Read the model definition and answer for the solid it produces. Units are mm, in the model's axes. Coordinates: 2 decimals unless noted, no trailing zeros. Loops run counter-clockwise (first coordinate to the right, second up) from the corner with the lowest first, then second, coordinate; pieces in that order, holes last. Notation, with made-up numbers: M 21.25,79 L 57.25,79 A13 cw 57.25,97 Z; hole C -7,11.25 d3. An arc over 180 degrees is marked long. One line per item, written item: value. Start each with the question number.
1. Flat-ended cylindrical pins translate along their axes: pin 1 (5 mm diameter, centred on y = 56, z = 7, fed in from +X); pin 2 (3 mm diameter, centred on x = 8.5, z = 8, fed in from +Y); pin 3 (3 mm diameter, centred on x = 22, z = 4, fed in from -Y); pin 4 (6 mm diameter, centred on x = 23.5, y = 21, fed in from -Z). Find the tip coordinate at first contact, or state that the pin passes through.
2. The part is cut by section A-A (z = 6.75). Write down the section's boundary in (x, y), then the cut area to 3 significant figures.
3. Consider probe 1 along X at (y, z) = (9.5, 7.25); probe 2 along Y at (x, z) = (23.5, 4.5); probe 3 along X at (y, z) = (19, 0.5). Determine where each line is inside the solid, lowest interval first.
```python
from build123d import *

# Parameters (mm, degrees)
EXTRUDE_1_DEPTH = 10
FILLET_1_R      = 0.5


with BuildPart() as part:
    # 草图1 → 凸台-拉伸1 (new body)
    with BuildSketch(Plane.XY):
        Polygon((0, 75), (37.5, 37.5), (0, 0), align=None)
    extrude(amount=EXTRUDE_1_DEPTH)

    # 圆角1
    fillet_1_edges = [part.edges().sort_by_distance(p)[0] for p in [
        (18.75, 56.25, 10),
        (18.75, 56.25, 0),
        (0, 37.5, 10),
        (18.75, 18.75, 0),
        (0, 37.5, 0),
        (0, 75, 5),
        (37.5, 37.5, 5),
        (0, 0, 5),
        (18.75, 18.75, 10),
    ]]
    fillet(fillet_1_edges, radius=FILLET_1_R)


solid = part.part
```
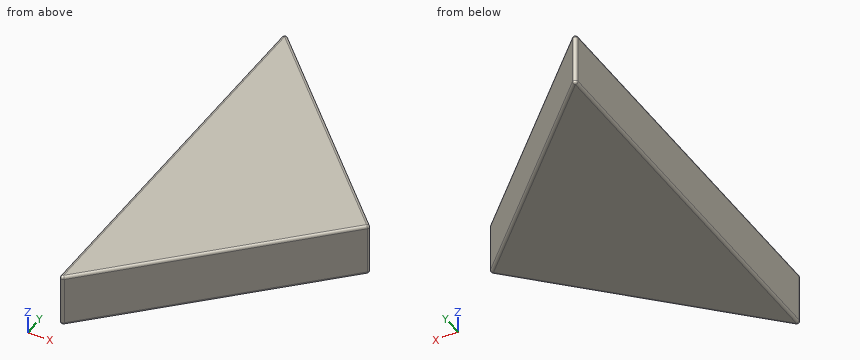
Answer block:
1. pin 1: stops at x = 21.5
1. pin 2: stops at y = 68
1. pin 3: stops at y = 20.5
1. pin 4: stops at z = 0
2. outline: M 0,1.21 A0.5 ccw 0.85,0.85 L 37.15,37.15 A0.5 ccw 37.15,37.85 L 0.85,74.15 A0.5 ccw 0,73.79 Z
2. area: 1,410 mm2
3. probe 1: x = 0 to 9.5
3. probe 2: y = 23.5 to 51.5
3. probe 3: x = 0 to 19
